Build history of the part. All positions in model axes, mm. Give positions to 0.01 mm unless a question says otherwise; leave off trailing zeros. Order: outer loops, then holes, each group sorted by start corner. A loop starts at its lowest first (then second) coordinate and runs counter-clockwise, first axis right, second up. Notation, with made-up numbers: (72.5, -38) - (102.5, -38) arc R5 cw to (102.5, -31) - close; hole circle Ø2 at (86, -40). An arc over 180 degrees is marked (long way). Use a Markdown table: item, result.
from build123d import *

# Parameters (mm, degrees)
F0_R     = 4.0005
F0_R_2   = 9.525
F0_R_3   = 7.9756
F1_DEPTH = 4.7752


with BuildPart() as f1:
    # F0 (on Front) → F1 (new body)
    with BuildSketch(Plane.XZ):
        with BuildLine():
            ThreePointArc((-6.35, 0), (-1.859872, 1.859872), (0, 6.35))
            Line((0, 6.35), (0, 247.65))
            ThreePointArc((0, 247.65), (-1.859872, 252.140128), (-6.35, 254))
            Line((-6.35, 254), (-95.25, 254))
            ThreePointArc((-95.25, 254), (-99.740128, 252.140128), (-101.6, 247.65))
            Line((-101.6, 247.65), (-101.6, 176.188146))
            ThreePointArc((-101.6, 176.188146), (-35.670644, 180.900035), (-1.27, 124.46))
            ThreePointArc((-1.27, 124.46), (-46.17483, 63.743695), (-117.379281, 88.9))
            Line((-117.379281, 88.9), (-247.65, 88.9))
            ThreePointArc((-247.65, 88.9), (-252.140128, 87.040128), (-254, 82.55))
            Line((-254, 82.55), (-254, 6.35))
            ThreePointArc((-254, 6.35), (-252.140128, 1.859872), (-247.65, 0))
            Line((-247.65, 0), (-6.35, 0))
        make_face()
        with Locations((-203.2, 38.1)):
            Circle(F0_R, mode=Mode.SUBTRACT)
        with Locations((-203.2, 76.2)):
            Circle(F0_R, mode=Mode.SUBTRACT)
        with Locations((-33.35242, 48.26)):
            Circle(F0_R_2, mode=Mode.SUBTRACT)
        with Locations((-88.9, 215.9)):
            Circle(F0_R, mode=Mode.SUBTRACT)
        with Locations((-38.1, 215.9)):
            Circle(F0_R, mode=Mode.SUBTRACT)
        with Locations((-7.62, 215.9)):
            Circle(F0_R, mode=Mode.SUBTRACT)
        with Locations((-33.35242, 48.26)):
            Circle(F0_R_2)
        with BuildLine():
            ThreePointArc((-1.27, 124.46), (-35.670644, 180.900035), (-101.6, 176.188146))
            Line((-101.6, 176.188146), (-101.6, 101.6))
            ThreePointArc((-101.6, 101.6), (-105.319744, 92.619744), (-114.3, 88.9))
            Line((-114.3, 88.9), (-117.379281, 88.9))
            ThreePointArc((-117.379281, 88.9), (-46.17483, 63.743695), (-1.27, 124.46))
        make_face()
        with Locations((-64.77, 124.46)):
            Circle(F0_R_3, mode=Mode.SUBTRACT)
    extrude(amount=F1_DEPTH)


solid = f1.part
1) Slice it at C-C (x = -203.2). Write the cut outline in (y, z), and give its area (3 significant figures).
Computed:
| item | result |
|---|---|
| outline | (-4.78, 0) - (0, 0) - (0, 34.1) - (-4.78, 34.1) - close; (-4.78, 42.1) - (0, 42.1) - (0, 72.2) - (-4.78, 72.2) - close; (-4.78, 80.2) - (0, 80.2) - (0, 88.9) - (-4.78, 88.9) - close |
| area | 348 mm² |
2) Slice it at A-A (x = -38.1). Write the cut outline in (y, z), and give its area (3 significant figures).
Computed:
| item | result |
|---|---|
| outline | (-4.78, 0) - (0, 0) - (0, 211.9) - (-4.78, 211.9) - close; (-4.78, 219.9) - (0, 219.9) - (0, 254) - (-4.78, 254) - close |
| area | 1,170 mm² |
3) Two-plate mould, pull along X, no slides. Class faces 1 (the cylindrical face through (-252.09, -2.35, 87.09)), 2 (the cylindrical face through (-199.505, -2.354, 74.668)), 3 (the cylindrical face through (-1.91, -2.35, 1.81)): +X half, -X half, draft (parallel to the pull), parting line (faces both ways), or undercut.
Computed:
| item | result |
|---|---|
| face 1 | -X half |
| face 2 | undercut |
| face 3 | +X half |
4) Pin check, flat tips, straight feed: P1, Ø9.5, axis at x = -64.77, z = 124.46, coming from the -Y side; P2, Ø1.5, axis at x = -31.5, z = 142.5, coming from the +Y side; P3, Ø2.5, axis at x = -175.5, y = -2, coming from the +Z side. Stop position of each tip, or through.
Computed:
| item | result |
|---|---|
| P1 | passes through |
| P2 | stops at y = 0 |
| P3 | stops at z = 88.9 |
5) Slice it at D-D (y = -2.15). Write the cut outline in (x, z), and give its area (3 significant figures).
Computed:
| item | result |
|---|---|
| outline | (-254, 6.35) arc R6.35 ccw to (-247.65, 0) - (-6.35, 0) arc R6.35 ccw to (0, 6.35) - (0, 247.65) arc R6.35 ccw to (-6.35, 254) - (-95.25, 254) arc R6.35 ccw to (-101.6, 247.65) - (-101.6, 101.6) arc R12.7 cw to (-114.3, 88.9) - (-247.65, 88.9) arc R6.35 ccw to (-254, 82.55) - close; hole circle Ø8 at (-203.2, 38.1); hole circle Ø8 at (-203.2, 76.2); hole circle Ø8 at (-88.9, 215.9); hole circle Ø15.95 at (-64.77, 124.46); hole circle Ø8 at (-38.1, 215.9); hole circle Ø8 at (-7.62, 215.9) |
| area | 38,900 mm² |
6) Wall check: line 1 (Z direction, x = -65.5, y = -2.4); line 2 (Z direction, x = -88.9, y = -3.25); line 3 (Z direction, x = -204, y = -3.6). Give the ranges that are in metal, low to high. Write a range as from..to.
Computed:
| item | result |
|---|---|
| line 1 | z = 0..116.52, 132.4..254 |
| line 2 | z = 0..211.9, 219.9..254 |
| line 3 | z = 0..34.18, 42.02..72.28, 80.12..88.9 |
7) Slice it at B-B (z = 124.46). Write the cut outline in (x, y).
Computed:
| item | result |
|---|---|
| outline | (-101.6, -4.78) - (-72.75, -4.78) - (-72.75, 0) - (-101.6, 0) - close; (-56.79, -4.78) - (0, -4.78) - (0, 0) - (-56.79, 0) - close |
